Input: part model. Units: mm. Frame: model coordinates. A direction names the side the tool comes from. Give positions to 0.01 mm unless a question says otherwise; leave off trailing zeros. Loops run counter-clockwise (first coordinate to the right, second up) from the corner with the lowest first, then second, coordinate; pieces in that order, holes last. Notation, with made-up numbers: (61, 14) -> (65, 14) arc R17 ccw to (65, 39) -> close; hole circle Ø2 at (-4.5, 62). An arc over 180 degrees is marked (long way). Use CSV: the item, a comma, the result in double quotes.
```python
from build123d import *

# Parameters (mm, degrees)
F0_R     = 250
F1_DEPTH = 12
F2_R     = 10
F3_DEPTH = 12
F5_DEPTH = 12


with BuildPart() as f1:
    # F0 (on Top) → F1 (new body)
    with BuildSketch(Plane.XY):
        Circle(F0_R)
    extrude(amount=F1_DEPTH)

    # F2 (on Top) → F3 (cut)
    with BuildSketch(Plane.XY):
        Circle(F2_R)
    extrude(amount=F3_DEPTH, mode=Mode.SUBTRACT)

    # F4 (on Top) → F5 (cut)
    with BuildSketch(Plane.XY):
        with BuildLine():
            Line((-17.189631, -242.445424), (-17.189631, 0))
            Line((-17.189631, 0), (-17.189631, 243.161663))
            ThreePointArc((-17.189631, 243.161663), (-244.387855, 0.35812), (-17.189631, -242.445424))
        make_face()
    extrude(amount=F5_DEPTH, mode=Mode.SUBTRACT)


solid = f1.part
```
1) Section query B-B (y = -19). Return loops of the section in (x, z).
From the geometry:
outline,"(-249.28, 0) -> (-243.62, 0) -> (-243.62, 12) -> (-249.28, 12) -> close; (-17.19, 0) -> (249.28, 0) -> (249.28, 12) -> (-17.19, 12) -> close"
2) Mould query, pull axis X, two halves, no side actions, for faces 1 (the cylindrical face through (-249.76, 10.99, 5.92)), 2 (the flat face through (-17.19, -3, 6)), 3 (the flat face through (108, 4, 0)). Classes: pulls with the +X half, pulls with the -X half, needs draft (parallel to the pull), parting line crosses it, or undercut.
From the geometry:
face 1,"parting line crosses it"
face 2,"undercut"
face 3,"needs draft"
3) Ray query, line 1 (Y direction, x = 0, z = 5); line 2 (X direction, y = -8, z = 1.5); line 3 (X direction, y = -224, z = 8). Return the intervals inside material, ascending.
From the geometry:
line 1,"y = -250 to -10, 10 to 250"
line 2,"x = -249.87 to -244.24, -17.19 to -6, 6 to 249.87"
line 3,"x = -111.01 to -95.27, -17.19 to 111.01"
4) Contact query for flat-ended pins moving along their axis: pin 1 (3 mm diameter, centred on y = 151, z = 4.5, fed in from -X); pin 2 (3 mm diameter, centred on x = 97.5, z = 4, fed in from -Y); pin 3 (5 mm diameter, centred on y = -68.5, z = 10, fed in from +X); pin 4 (8 mm diameter, centred on x = -24.5, y = 31, fed in from +Z). Output: stop coordinate, or through.
From the geometry:
pin 1,"stops at x = -200.37"
pin 2,"stops at y = -230.83"
pin 3,"stops at x = 241.13"
pin 4,"passes through"
5) Section query C-C (z = 10). Return loops of the section in (x, y), then the cut area to 3 significant figures.
From the geometry:
outline,"circle Ø500 at (0, 0); hole (-17.19, -242.45) -> (-17.19, 243.16) arc R243.34 ccw to start; hole circle Ø20 at (0, 0)"
area,"111,000 mm^2"
6) Reachability of faces 4 (the cylindrical face through (-244.334, 5.483, 5.916)), 5 (the flat face through (108, 4, 12)) from +Z, -Z, +X, -X, +Y, -Y: full face, straight path, thin tool, end or side. Return the list, or none.
From the geometry:
face 4,"+Z, -Z"
face 5,"+Z, +X, -X, +Y, -Y"
7) Section query A-A (x = -47). Return loops of the section in (y, z), then the cut area to 3 significant figures.
From the geometry:
outline,"(-245.54, 0) -> (-238.6, 0) -> (-238.6, 12) -> (-245.54, 12) -> close; (239.32, 0) -> (245.54, 0) -> (245.54, 12) -> (239.32, 12) -> close"
area,"158 mm^2"
8) Section query D-D (x = 60). Return loops of the section in (y, z), then the cut area to 3 significant figures.
From the geometry:
outline,"(-242.69, 0) -> (242.69, 0) -> (242.69, 12) -> (-242.69, 12) -> close"
area,"5,820 mm^2"
